Solid Edge part; units mm, degrees
sketch "Sketch1" plane through (0, 0, 0) normal (0, -1, 0) x (1, 0, 0)
  line L0 (21.2, 4.4667) -> (41.2, 4.4667)
  line L1 (41.2, 4.4667) -> (41.2, 44.4667)
  line L2 (41.2, 44.4667) -> (21.2, 44.4667)
  line L3 (21.2, 44.4667) -> (21.2, 4.4667)
  dimension "D1" = 21.2
  dimension "D2" = 41.2
extrude "Protrusion1" add sketch "Sketch1" against normal blind 15
sketch "Sketch2" plane through (31.2, 0, 24.4667) normal (0, -1, 0) x (1, 0, 0)
  circle A0 centre (0, 10) radius 6
extrude "ExtrudedCutout_1" cut sketch "Sketch2" against normal blind 10
sketch "Sketch3" plane through (21.2, 7.5, 24.4667) normal (-1, 0, 0) x (0, -1, 0)
  line L0 (7.5, 13) -> (2.5, 13)
  arc A0 (2.5, 13) -> (2.5, 7) centre (2.5, 10) ccw
  line L1 (2.5, 7) -> (7.5, 7)
  line L2 (7.5, 13) -> (7.5, 7)
  dimension "D1" = 7.5
extrude "Cutout1" cut sketch "Sketch3" against normal through all
sketch "Sketch4" plane through (31.2, 15, 24.4667) normal (0, 1, 0) x (-1, 0, 0)
  line L0 (-10, 20) -> (-4, 20)
  line L1 (-4, 20) -> (-4, -20)
  line L2 (-4, -20) -> (-10, -20)
  line L3 (-10, -20) -> (-10, 20)
  dimension "D1" = 10
extrude "Cutout2" cut sketch "Sketch4" against normal through all
sketch "Sketch5" plane through (28.2, 7.5, 4.4667) normal (0, 0, -1) x (1, 0, 0)
  line L0 (5.4019, 7.5) -> (5.4019, 2.5)
  arc A0 (5.4019, 2.5) -> (-0.5981, 2.5) centre (2.4019, 2.5) cw
  line L1 (-0.5981, 2.5) -> (-0.5981, 7.5)
  line L2 (5.4019, 7.5) -> (-0.5981, 7.5)
  dimension "D1" = 0.5981
  dimension "D2" = 5.4019
extrude "Cutout3" cut sketch "Sketch5" against normal up to next
sketch "Sketch6" plane through (28.2, 15, 24.4667) normal (0, 1, 0) x (-1, 0, 0)
  line L0 (-7, -20) -> (7, -20)
  line L1 (7, -20) -> (7, -1)
  line L2 (7, -1) -> (-7, -1)
  line L3 (-7, -1) -> (-7, -20)
  dimension "D1" = 7
extrude "Cutout4" cut sketch "Sketch6" against normal up to next
sketch "Sketch7" plane through (28.2, 15, 33.9667) normal (0, 1, 0) x (-1, 0, 0)
  line L0 (-39.04, 20.5) -> (-39.04, -19.5)
  line L1 (-39.04, -19.5) -> (50.96, -19.5)
  line L2 (50.96, 20.5) -> (50.96, -19.5)
  line L3 (-39.04, 20.5) -> (50.96, 20.5)
  dimension "D1" = 39.04
  dimension "D2" = 39.04
  dimension "D3" = 50.96
extrude "ExtrudedProtrusion_2" add sketch "Sketch7" along normal blind 3
sketch "Sketch8" plane through (19.24, 18, 34.4667) normal (0, 1, 0) x (-1, 0, 0)
  circle A0 centre (-43, 15) radius 1.65
  circle A1 centre (37, -15) radius 1.65
  dimension "D1" = 43
extrude "Cutout5" cut sketch "Sketch8" against normal through all
sketch "Sketch9" plane through (19.24, 18, 34.4667) normal (0, 1, 0) x (-1, 0, 0)
  circle A0 centre (-43, 15) radius 3.55
  circle A1 centre (37, -15) radius 3.55
extrude "ExtrudedCutout_9" cut sketch "Sketch9" against normal blind 0.5
For this review, take the finished solid that the model builds, in its own axes (mm). A direction names the side the tool comes from. Coordinates: 2 decimals unless noted, no trailing zeros. Order: outer loops, then holes, each group sorted by start corner. A loop starts at its lowest first (then second) coordinate and runs counter-clockwise, first axis right, second up. Notation, with made-up numbers: (40, 35) -> (46, 35) arc R23 cw to (46, 49) -> close; hole circle Ø4 at (12, -26). An arc over 180 degrees is marked (long way). Use CSV: the item, a comma, the result in double quotes. Start each with the question number.
Item 1: We need section D-D, the plane x = 40. Give the boundary of the cut face in (y, z).
Item 2: For faces 1 (the face through (-17.298, 17.754, 22.986)), 2 (the face through (30, 10, 35)), 3 (the face through (27.602, 3, 27)), 4 (the face through (24, 2, 37.467)), list the 3-axis set-ups (+Z, -Z, +X, -X, +Y, -Y) from which the entire face can be reached by the end or side of a thin tool; tool diameter is ignored.
Item 3: We need section A-A, the plane x = -17.76. Give the boundary of the cut face in (y, z).
Item 4: Insertion check: pin 1 (7.5 mm diameter, centred on y = 8, z = 38, fed in from +X); pin 2 (10 mm diameter, centred on y = 3, z = 30, fed in from -X); pin 3 (9 mm diameter, centred on x = 62.24, z = 49.47, fed in from -Y). Each pin has a flat end and moves straight along its axis. Give the tip position at first contact, or say it passes through.
Item 5: We need section B-B, the plane z = 41.5. Give the boundary of the cut face in (x, y), then the cut area to 3 significant figures.
Item 6: Wall thickness on probe 1 along Z at (x, y) = (-17.76, 17.75); probe 2 along Z at (x, y) = (-17.76, 15.95); probe 3 along Y at (x, z) = (-14, 21): over which ranges is each line inside the solid? List them lowest first.
Item 7: Draft analysis for pull direction X (two halves, no side actions). For faces 5 (the face through (23.6, 8, 34.5)), 6 (the face through (21.2, 9, 34)), 7 (the face through (65.06, 17.75, 47.31)), 8 (the face through (28.239, 6.041, 39.685)), state which applies: pulls with the +X half, pulls with the -X half, needs draft (parallel to the pull), parting line crosses it, or undercut.
Item 8: We need section C-C, the plane y = 2.25. Give the boundary of the cut face in (x, z), then the cut area to 3 significant figures.
Derived:
1,outline,"(15, 14.47) -> (18, 14.47) -> (18, 54.47) -> (15, 54.47) -> close"
2,face 1,"+Y"
2,face 2,"-Y"
2,face 3,"-Z, -Y"
2,face 4,"+X, -X, -Y"
3,outline,"(15, 14.47) -> (18, 14.47) -> (18, 15.92) -> (17.5, 15.92) -> (17.5, 17.82) -> (15, 17.82) -> close; (15, 21.12) -> (17.5, 21.12) -> (17.5, 23.02) -> (18, 23.02) -> (18, 54.47) -> (15, 54.47) -> close"
4,pin 1,"stops at x = 35.2"
4,pin 2,"stops at x = 21.2"
4,pin 3,"stops at y = 15"
5,outline,"(-22.76, 15) -> (21.2, 15) -> (21.2, 0) -> (35.2, 0) -> (35.2, 15) -> (67.24, 15) -> (67.24, 18) -> (-22.76, 18) -> close"
5,area,"480 mm^2"
6,probe 1,"z = 14.47 to 15.92, 23.02 to 54.47"
6,probe 2,"z = 14.47 to 17.82, 21.12 to 54.47"
6,probe 3,"y = 15 to 18"
7,face 5,"needs draft"
7,face 6,"pulls with the -X half"
7,face 7,"undercut"
7,face 8,"undercut"
8,outline,"(21.2, 23.47) -> (27.6, 23.47) -> (27.6, 29.67) arc R6 cw to (26, 31.47) -> (21.2, 31.47) -> close; (21.2, 37.47) -> (26, 37.47) arc R6 cw to (35.2, 38.94) -> (35.2, 44.47) -> (21.2, 44.47) -> close; (33.6, 23.47) -> (35.2, 23.47) -> (35.2, 29.99) arc R6 cw to (33.6, 28.97) -> close"
8,area,"136 mm^2"
